from build123d import *

# Parameters (mm, degrees)
F1_DEPTH = 15
F2_DEPTH = 125
F4_DEPTH = 15


with BuildPart() as f1:
    # F0 (on Front) → F1 (new body)
    with BuildSketch(Plane.XZ):
        with BuildLine():
            Line((-5, 0), (0, 0))
            Line((0, 0), (0, 5))
            Line((0, 5), (5, 5))
            Line((5, 5), (10, 5))
            Line((10, 5), (10, 0))
            Line((10, 0), (15, 0))
            ThreePointArc((15, 0), (5, 10), (-5, 0))
        make_face()
        with BuildLine():
            ThreePointArc((5, 5), (1.4644660941, 3.5355339059), (0, 0))
            Line((0, 0), (10, 0))
            ThreePointArc((10, 0), (8.5355339059, 3.5355339059), (5, 5))
        make_face()
        with BuildLine():
            Line((0, 5), (0, 0))
            ThreePointArc((0, 0), (1.4644660941, 3.5355339059), (5, 5))
            Line((5, 5), (0, 5))
        make_face()
        with BuildLine():
            ThreePointArc((5, 5), (8.5355339059, 3.5355339059), (10, 0))
            Line((10, 0), (10, 5))
            Line((10, 5), (5, 5))
        make_face()
    extrude(amount=F1_DEPTH)

    # F0 (on Front) + F1_face (on face) → F2 (join)
    with BuildSketch(Plane.XZ):
        with BuildLine():
            Line((-5, 0), (0, 0))
            Line((0, 0), (0, 5))
            Line((0, 5), (5, 5))
            Line((5, 5), (10, 5))
            Line((10, 5), (10, 0))
            Line((10, 0), (15, 0))
            ThreePointArc((15, 0), (5, 10), (-5, 0))
        make_face()
        with BuildLine():
            ThreePointArc((5, 5), (8.5355339059, 3.5355339059), (10, 0))
            Line((10, 0), (10, 5))
            Line((10, 5), (5, 5))
        make_face()
        with BuildLine():
            Line((0, 5), (0, 0))
            ThreePointArc((0, 0), (1.4644660941, 3.5355339059), (5, 5))
            Line((5, 5), (0, 5))
        make_face()
    with BuildSketch(Plane(origin=(5, 0, 4.2441318158), x_dir=(1, 0, 0), z_dir=(0, 1, 0))):
        with BuildLine():
            Line((10, 4.2441318158), (-10, 4.2441318158))
            ThreePointArc((-10, 4.2441318158), (0, -5.7558681842), (10, 4.2441318158))
        make_face()
    extrude(amount=-F2_DEPTH, dir=(0, -1, 0))

    # F3 (on face) → F4 (cut)
    with BuildSketch(Plane(origin=(0, 125, 0), x_dir=(-1, 0, 0), z_dir=(0, 1, 0))):
        with BuildLine():
            Line((-12, 1.5), (2, 1.5))
            ThreePointArc((2, 1.5), (-5, 8.5), (-12, 1.5))
        make_face()
    extrude(amount=-F4_DEPTH, mode=Mode.SUBTRACT)


solid = f1.part
Input: part model. Units: mm. Frame: model coordinates. A direction names the side the tool comes from. Coordinates: 2 decimals unless noted, no trailing zeros. Loops run counter-clockwise (first coordinate to the right, second up) from the corner with the lowest first, then second, coordinate; pieces in that order, holes last.
(1) Material intervals for probe 1 along Y at (x, z) = (1.25, 4.75); probe 2 along X at (y, z) = (112.5, 7); probe 3 along X at (y, z) = (99, 0.75), sorted ascending.
(2) Set-up query: faces 4 (the face through (5, -15, 4)), 5 (the face through (5, 118, 1.5)). Return all of +Z, -Z, +X, -X, +Y, -Y with unobstructed straight access to the full face (end or side cutting, diameter ignored); none if empty.
(3) Section A-A on x = 5. Return the cut outline in (y, z), then the cut area to 4 significant figures.
(4) First-contact query: pin 1 Ø7 at (x, y) = (3.5, 117.5) entering from +Z; pin 2 Ø4 at (y, z) = (67, 7.5) entering from +X; pin 3 Ø1 at (y, z) = (36.5, 3) entering from -X; pin 4 Ø3.5 at (x, z) = (7.5, 3.5) entering from +Y. Flat tips, straight axial feed; report the tip coordinate or a pass-through.
(5) Section B-B on z = 7. Return the cut outline in (x, y).
(6) Pull-direction query (Z, two-part tool) for faces 1 (the face through (4.85, 117.6, 8.5)), 2 (the face through (5, 125, 1)), 3 (the face through (5, 54, 0)); classes: released by +Z, released by -Z, zero draft, split by the parting line, or undercut.
(7) Section C-C on y = 82.5. Return the cut outline in (x, z), then the cut area to 3 significant figures.
Data:
1. probe 1: y = -15 to 110
1. probe 2: x = -2.14 to 0.67, 9.33 to 12.14
1. probe 3: x = -4.97 to 14.97
2. face 4: +Z, -Z, +X, -X, -Y
2. face 5: +Y
3. outline: (-15, 0) - (125, 0) - (125, 1.5) - (110, 1.5) - (110, 8.5) - (125, 8.5) - (125, 10) - (-15, 10) - close
3. area: 1,295 mm2
4. pin 1: stops at z = 10
4. pin 2: stops at x = 13.35
4. pin 3: stops at x = -4.68
4. pin 4: stops at y = 110
5. outline: (-2.14, -15) - (12.14, -15) - (12.14, 125) - (9.33, 125) - (9.33, 110) - (0.67, 110) - (0.67, 125) - (-2.14, 125) - close
6. face 1: undercut
6. face 2: zero draft
6. face 3: released by -Z
7. outline: (-5, 0) - (15, 0) arc R10 ccw to start
7. area: 157 mm2
